```python
from build123d import *

# Parameters (mm, degrees)
BOSS_EXTRUDE1_DEPTH = 12.8
SKETCH2_W           = 65
SKETCH2_H           = 80
CUT_EXTRUDE1_DEPTH  = 5
SKETCH3_R           = 2.5
BOSS_EXTRUDE2_DEPTH = 65
BOSS_EXTRUDE3_START = 65
BOSS_EXTRUDE3_DEPTH = 65


with BuildPart() as part:
    # Sketch1 → Boss-Extrude1 (new body)
    with BuildSketch(Plane(origin=(0, 0, 0), x_dir=(1, 0, 0), z_dir=(0, 1, 0))):
        with BuildLine():
            Line((-32.5, -43), (32.5, -43))
            ThreePointArc((32.5, -43), (34.621320344, -42.121320344), (35.5, -40))
            Line((35.5, -40), (35.5, 40))
            ThreePointArc((35.5, 40), (34.621320344, 42.121320344), (32.5, 43))
            Line((32.5, 43), (-32.5, 43))
            ThreePointArc((-32.5, 43), (-34.621320344, 42.121320344), (-35.5, 40))
            Line((-35.5, 40), (-35.5, -40))
            ThreePointArc((-35.5, -40), (-34.621320344, -42.121320344), (-32.5, -43))
        make_face()
    extrude(amount=BOSS_EXTRUDE1_DEPTH)

    # Sketch2 → Cut-Extrude1 (cut)
    with BuildSketch(Plane(origin=(0, 12.8, 0), x_dir=(1, 0, 0), z_dir=(0, 1, 0))):
        Rectangle(SKETCH2_W, SKETCH2_H)
    extrude(amount=-CUT_EXTRUDE1_DEPTH, mode=Mode.SUBTRACT)

    # Sketch3 → Boss-Extrude2 (add)
    with BuildSketch(Plane(origin=(-32.5, 0, 0), x_dir=(0, 0, -1), z_dir=(1, 0, 0))):
        with Locations((0, 9.096601027)):
            Circle(SKETCH3_R)
    extrude(amount=BOSS_EXTRUDE2_DEPTH)

    # Sketch4 → Boss-Extrude3 (add)
    with BuildSketch(Plane.ZY.offset(-32.5).offset(BOSS_EXTRUDE3_START)):
        with BuildLine():
            Line((-2.454816759, 8.623447059), (-14.48112221, 8.623447059))
            Line((-14.48112221, 8.623447059), (-28.991763091, 7.8))
            Line((-28.991763091, 7.8), (-2.137481176, 7.8))
            ThreePointArc((-2.137481176, 7.8), (-2.332770101, 8.197610675), (-2.454816759, 8.623447059))
        make_face()
        with BuildLine():
            Line((2.452414649, 8.611150321), (14.48112221, 8.623447059))
            Line((14.48112221, 8.623447059), (28.991763091, 7.8))
            Line((28.991763091, 7.8), (2.137481176, 7.8))
            ThreePointArc((2.137481176, 7.8), (2.330510058, 8.191767966), (2.452414649, 8.611150321))
        make_face()
    extrude(amount=-BOSS_EXTRUDE3_DEPTH)


solid = part.part
```
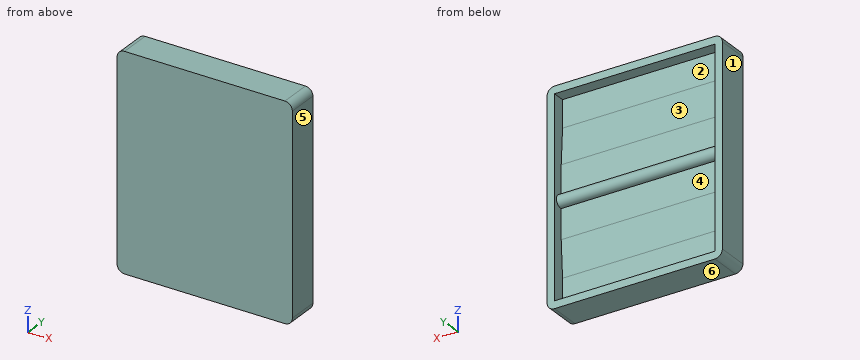
CAD build for the part. Positions are in the model's coordinates, mm. Face numbers are marked on the shaded views. A direction names the side the tool comes from. Coordinates: 2 decimals unless noted, no trailing zeros. Order: outer loops, then holes, each group sorted by start corner. A loop starts at its lowest first (then second) coordinate and runs counter-clockwise, first axis right, second up.
(1) Drill centre lines: L1, parallel to Z at x = -13, y = 9; L2, parallel to Y at x = 13.5, z = 10; L3, parallel to X at y = 11.75, z = -23.5. Where is each one in solid material? Low to high.
Solution:
L1: z = -43 to -40, -2.5 to 2.5, 40 to 43
L2: y = 0 to 8.62
L3: x = -35.5 to -32.5, 32.5 to 35.5
(2) Saw through at B-B, the plane z = 35.5. Write the cut outline in (x, y).
Solution:
outline: (-35.5, 0) - (35.5, 0) - (35.5, 12.8) - (32.5, 12.8) - (32.5, 7.8) - (-32.5, 7.8) - (-32.5, 12.8) - (-35.5, 12.8) - close
(3) Saw through at D-D, the plane z = -7. Write the cut outline in (x, y), and give its area (3 significant figures).
Solution:
outline: (-35.5, 0) - (35.5, 0) - (35.5, 12.8) - (32.5, 12.8) - (32.5, 8.62) - (-32.5, 8.62) - (-32.5, 12.8) - (-35.5, 12.8) - close
area: 637 mm2
(4) Pin check, flat tips, straight feed: pin 1 Ø13 at (x, z) = (7.5, -8.5) entering from +Y; pin 2 Ø12 at (x, z) = (-8.5, -32) entering from +Y; pin 3 Ø5 at (x, z) = (22, 9.5) entering from +Y. Stop position of each tip, or through.
Solution:
pin 1: stops at y = 10.6
pin 2: stops at y = 7.97
pin 3: stops at y = 8.62
(5) Saw through at C-C, the plane y = 10.25. Write the cut outline in (x, z).
Solution:
outline: (-35.5, -40) arc R3 ccw to (-32.5, -43) - (32.5, -43) arc R3 ccw to (35.5, -40) - (35.5, 40) arc R3 ccw to (32.5, 43) - (-32.5, 43) arc R3 ccw to (-35.5, 40) - close; hole (-32.5, -40) - (32.5, -40) - (32.5, -2.22) - (-32.5, -2.22) - close; hole (-32.5, 2.22) - (32.5, 2.22) - (32.5, 40) - (-32.5, 40) - close
(6) Mould opens along Z. For the marked faces 3, 4, 5 and 6 say: released by +Z, released by -Z, zero draft, split by the parting line, or undercut.
Solution:
face 3: undercut
face 4: undercut
face 5: zero draft
face 6: released by -Z
(7) Saw through at A-A, the plane x = 25. Write the cut outline in (y, z).
Solution:
outline: (0, -43) - (12.8, -43) - (12.8, -40) - (7.8, -40) - (7.8, -28.99) - (8.62, -14.48) - (8.62, -2.45) arc R2.5 ccw (long way) to (8.61, 2.45) - (8.62, 14.48) - (7.8, 28.99) - (7.8, 40) - (12.8, 40) - (12.8, 43) - (0, 43) - close
(8) Which spindle directions (+Z, -Z, +X, -X, +Y, -Y) get a long thin tool onto all of the face, cutting with end or side? Do the marked faces 1 and 2. Say none if no direction does.
Solution:
face 1: +Z, -Z, -X, +Y, -Y
face 2: +Y
